```python
from build123d import *

# Parameters (mm, degrees)
F1_DEPTH = 10
F3_DEPTH = 10
F4_R     = 5
F6_D     = 3.3
F6_DEPTH = 10
F6_TIP   = 0.9914200214
F8_DEPTH = 2


with BuildPart() as f1:
    # F0 (on Right) → F1 (new body)
    with BuildSketch(Plane.YZ):
        Polygon((0, 22.2580076184), (0, 0), (93.8056360581, 0), (73.2522689977, 95.1130465462), (33.0475914831, 95.1130465462), align=None)
        Polygon((68.4103418893, 89.1130465462), (85.9383917163, 8), (5.9322550672, 8), (5.9322550672, 20.8114475514), (36.9143720826, 89.1130465462), align=None, mode=Mode.SUBTRACT)
    extrude(amount=F1_DEPTH)

    # F2 (on face) → F3 (join)
    with BuildSketch(Plane(origin=(0, 0, 0), x_dir=(0, -1, 0), z_dir=(-1, 0, 0))):
        Polygon((-85.9383917163, 8), (-92.0768833533, 8), (-93.8056360581, 0), (0, 0), (0, 8), (-5.9322550672, 8), align=None)
    extrude(amount=F3_DEPTH)

    # F4
    f4_edges = [f1.edges().sort_by_distance(p)[0] for p in [
        (-10, 92.94126, 4),
        (-10, 0, 4),
        (5, 73.252269, 95.113047),
    ]]
    fillet(f4_edges, radius=F4_R)

    # F6
    with Locations(Plane(origin=(0, -8.3734748609, 3.7982709305), x_dir=(1, 0, 0), z_dir=(0, -0.9106879866, 0.4130948935))):
        with Locations((5, 89.7701001437), (5, 40.2701001437)):
            Hole(F6_D / 2, depth=F6_DEPTH)
            with Locations((0, 0, -(F6_DEPTH + F6_TIP / 2))):  # 118° drill point
                Cone(0, F6_D / 2, F6_TIP, mode=Mode.SUBTRACT)

    # F7 (on face) → F8 (cut)
    with BuildSketch(Plane(origin=(0, -2.9093469413, 1.3197015692), x_dir=(-1, 0, 0), z_dir=(0, 0.9106879866, -0.4130948935))):
        Polygon((-7.75, 41.857813384), (-7.75, 38.6823869034), (-5, 37.0946736632), (-2.25, 38.6823869034), (-2.25, 41.857813384), (-5, 43.4455266242), align=None)
        Polygon((-7.75, 91.357813384), (-7.75, 88.1823869034), (-5, 86.5946736632), (-2.25, 88.1823869034), (-2.25, 91.357813384), (-5, 92.9455266242), align=None)
    extrude(amount=-F8_DEPTH, mode=Mode.SUBTRACT)


solid = f1.part
```
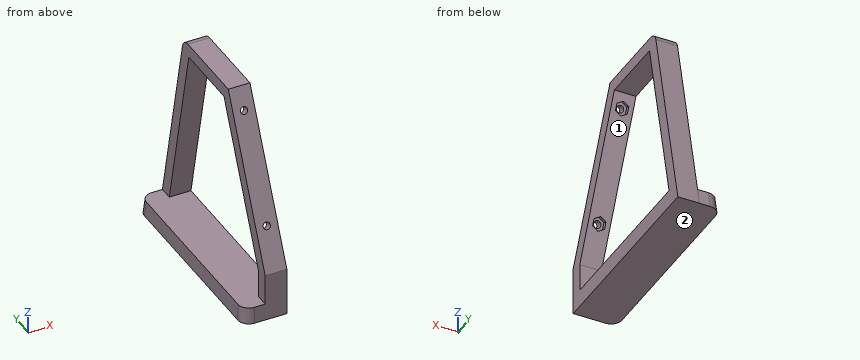
CAD build for the part. Positions are in the model's coordinates, mm. Face numbers are marked on the shaded views. A direction names the side the tool comes from. Coordinates: 2 decimals unless noted, no trailing zeros. Write each loop counter-clockwise with the first axis right and the second up, starting at its lowest first coordinate (ties: lowest second). Pieces come first, ordered by that corner, then holes.
(1) Cut at A-A, the plane y = 38.5. List the corners of the cut face in (x, z).
(2) Cut at B-B, the plane z = 17.5. List the corners of the cut face in (x, y).
(3) Cut at C-C, the plane x = -8. List the corners of the cut face in (y, z), and give its area (3 significant figures).
(4) 3-axis set-ups, long thin cutter, end or side, ignore diameter. For the marked faces 1 and 2: which of +Z, -Z, +X, -X, +Y, -Y reach the whole face in a straight line?
(5) Drill centre lines: probe 1 along Z at (x, y) = (6.75, 66.5); probe 2 along Z at (x, y) = (-6, 81); probe 3 along Y at (x, z) = (5, 30.5). Where is each one in solid material? Low to high.
(6) Flat gauge pins, fed straight in: pin 1 (3.5 mm diameter, centred on y = 12.5, z = 38.5, fed in from -X); pin 2 (12 mm diameter, centred on x = -6.5, y = 30.5, fed in from +Z); pin 3 (8 mm diameter, centred on x = 4.5, z = 13.5, fed in from +Y). Where does each tip first touch, or does it go through?
Geometry says:
1. outline: (-10, 0) - (10, 0) - (10, 8) - (-10, 8) - close; (0, 89.11) - (10, 89.11) - (10, 95.11) - (0, 95.11) - close
2. outline: (0, 0) - (10, 0) - (10, 5.93) - (0, 5.93) - close; (0, 83.89) - (10, 83.89) - (10, 90.02) - (0, 90.02) - close
3. outline: (1, 0) - (92.78, 0) - (91.05, 8) - (1, 8) - close
3. area: 727 mm2
4. face 1: +X, -X
4. face 2: -Z, +X, -X, +Y, -Y
5. probe 1: z = 0 to 8, 89.11 to 95.11
5. probe 2: z = 0 to 8
5. probe 3: y = 3.74 to 10.33, 81.08 to 87.21
6. pin 1: stops at x = 0
6. pin 2: stops at z = 8
6. pin 3: stops at y = 91.75
